The figure shows three views and two pictorial views of one solid part (mm, origin at its lowest corner). Answer the questions. A direction names the side the tool comes from. Give positions to 0.01 mm unless a question says otherwise; leave off trailing zeros. Order: outer loops, then holes, each group sorted by start corner. A loop starts at its lowest first (then second) coordinate and runs counter-clockwise, first axis right, second up. Notation, with made-up numbers: M 69.25,50 L 84.25,50 A14 ccw 84.25,76 Z; hole C 21,50.25 d7. An arc over 180 degrees is marked long. One line per item, written item: value.
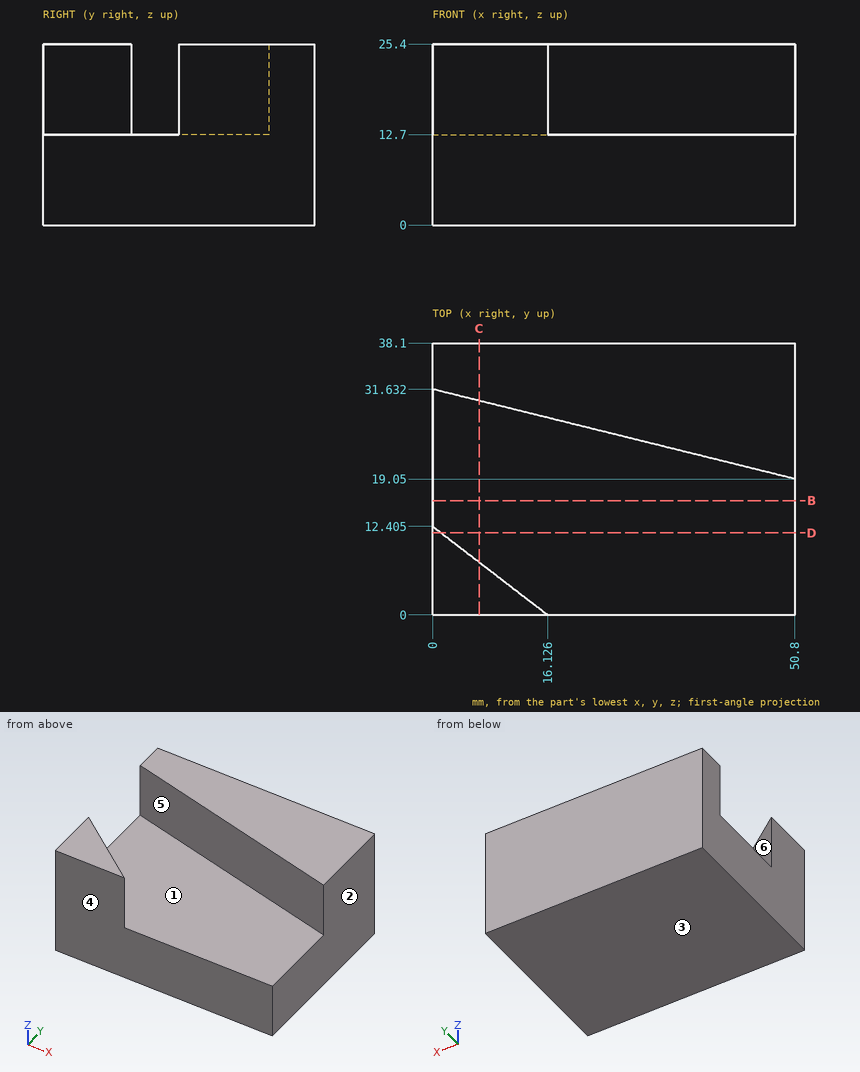
1) Find section C-C, the plane x = 6.5. Write down the section's boundary in (y, z) (1 decimal).
Reported:
outline: M 0,0 L 38.1,0 L 38.1,25.4 L 30,25.4 L 30,12.7 L 7.4,12.7 L 7.4,25.4 L 0,25.4 Z
2) Determine the mould class of the marked faces 3, 4, 5 and 6 for opening direction Y: +Y half, -Y half, draft (parallel to the pull), parting line (faces both ways), or undercut.
Reported:
face 3: draft
face 4: -Y half
face 5: undercut
face 6: undercut
3) Consider probe 1 along Z at (x, y) = (28, 8.5); probe 2 along Y at (x, z) = (7.5, 24.75) (1 decimal); probe 3 along X at (y, z) = (5.5, 18.25) (1 decimal). Determine where each line is inside the solid, lowest interval first.
Reported:
probe 1: z = 0 to 12.7
probe 2: y = 0 to 6.6, 29.8 to 38.1
probe 3: x = 0 to 9
4) Each of these flat-tipped pins is pushed along its axis until it touches: pin 1 Ø3 at (x, y) = (17, 7.5) entering from +Z; pin 2 Ø1.5 at (x, z) = (31, 20.5) entering from -Y; pin 3 Ø2 at (x, z) = (42.5, 19.5) entering from -Y. Where does it stop, or does it pass through?
Reported:
pin 1: stops at z = 12.7
pin 2: stops at y = 23.77
pin 3: stops at y = 20.86
5) Which of the six approach directions +Z, -Z, +X, -X, +Y, -Y give full straight-line access (tool end or side, diameter ignored) to the marked faces 1 and 2?
Reported:
face 1: +Z
face 2: +Z, -Z, +X, +Y, -Y
6) Find section B-B, the plane y = 16. Write down the section's boundary in (x, z).
Reported:
outline: M 0,0 L 50.8,0 L 50.8,12.7 L 0,12.7 Z
7) Find section D-D, the plane y = 11.5. Write down the section's boundary in (x, z).
Reported:
outline: M 0,0 L 50.8,0 L 50.8,12.7 L 1.18,12.7 L 1.18,25.4 L 0,25.4 Z
